```python
from build123d import *

# Parameters (mm, degrees)
SKETCH2_W           = 100
SKETCH2_H           = 50
BOSS_EXTRUDE1_DEPTH = 25
CUT_EXTRUDE1_DEPTH  = 9
CUT_EXTRUDE2_DEPTH  = 6.4
SKETCH8_W           = 6
SKETCH8_H           = 6
CUT_EXTRUDE3_DEPTH  = 6
SKETCH9_W           = 5
SKETCH9_H           = 5
CUT_EXTRUDE4_DEPTH  = 5


with BuildPart() as part:
    # Sketch2 → Boss-Extrude1 (new body)
    with BuildSketch(Plane(origin=(0, 0, 0), x_dir=(1, 0, 0), z_dir=(0, 1, 0))):
        Rectangle(SKETCH2_W, SKETCH2_H)
    extrude(amount=-BOSS_EXTRUDE1_DEPTH)

    # Sketch3 → Cut-Loft4 section 0
    with BuildSketch(Plane(origin=(0, 0, 0), x_dir=(1, 0, 0), z_dir=(0, 1, 0))):
        with BuildLine():
            Line((-45, 20), (45, 20))
            Line((45, 20), (45, -20))
            Line((45, -20), (-45, -20))
            Line((-45, -20), (-45, 20))
        make_face()
    # Sketch4 → Cut-Loft4 section 1
    with BuildSketch(Plane.XZ.offset(25)):
        with BuildLine():
            Line((-5, 5), (5, 5))
            Line((5, 5), (5, -5))
            Line((5, -5), (-5, -5))
            Line((-5, -5), (-5, 5))
        make_face()
    loft(mode=Mode.SUBTRACT)

    # Sketch5 → Cut-Extrude1 (cut)
    with BuildSketch(Plane(origin=(0, 0, -25), x_dir=(-1, 0, 0), z_dir=(0, 0, -1))):
        Polygon((0, -8), (3.2, -8), (3.2, -25), (-3.2, -25), (-3.2, -8), align=None)
    extrude(amount=-CUT_EXTRUDE1_DEPTH, mode=Mode.SUBTRACT)

    # Sketch6 → Cut-Extrude2 (cut)
    with BuildSketch(Plane(origin=(-3.2, 0, 0), x_dir=(0, 0, -1), z_dir=(1, 0, 0))):
        Polygon((16, -25), (5.785369477, -25), (16, -8), align=None)
    extrude(amount=CUT_EXTRUDE2_DEPTH, mode=Mode.SUBTRACT)

    # Sketch8 → Cut-Extrude3 (cut)
    with BuildSketch(Plane.XZ.offset(25)):
        with Locations((-45, 20)):
            Rectangle(SKETCH8_W, SKETCH8_H)
        with Locations((45, 20)):
            Rectangle(SKETCH8_W, SKETCH8_H)
    extrude(amount=-CUT_EXTRUDE3_DEPTH, mode=Mode.SUBTRACT)

    # Sketch9 → Cut-Extrude4 (cut)
    with BuildSketch(Plane(origin=(0, 0, 0), x_dir=(1, 0, 0), z_dir=(0, 1, 0))):
        with Locations((47.5, -22.5)):
            Rectangle(SKETCH9_W, SKETCH9_H)
        with Locations((-47.5, -22.5)):
            Rectangle(SKETCH9_W, SKETCH9_H)
        with Locations((-47.5, 22.5)):
            Rectangle(SKETCH9_W, SKETCH9_H)
        with Locations((47.5, 22.5)):
            Rectangle(SKETCH9_W, SKETCH9_H)
    extrude(amount=-CUT_EXTRUDE4_DEPTH, mode=Mode.SUBTRACT)


solid = part.part
```
Build history of the part. All positions in model axes, mm. A direction names the side the tool comes from. Coordinates: 2 decimals unless noted, no trailing zeros. Order: outer loops, then holes, each group sorted by start corner. A loop starts at its lowest first (then second) coordinate and runs counter-clockwise, first axis right, second up. Notation, with made-up numbers: (66, 7.25) -> (118, 7.25) arc R9 ccw to (118, 22.25) -> close; hole circle Ø2 at (57.25, 35). An arc over 180 degrees is marked (long way). Answer in a Markdown table with one row per item. Add a question column.
Q1. Wall check: line 1 along X through (y, z) = (-23.25, 21.5); line 2 along X through (y, z) = (-5.25, 14.5); line 3 along X through (y, z) = (-1.75, 20.5). Give the ranges that are in metal, low to high. Write a range as [from, to].
Q2. Mould opens along Z. For faces 1 (the face through (-45, -22, 17)), 2 (the face through (47, -5, -23)), 3 (the face through (45, -22, 23)), 4 (the face through (-1, -7, -25)) say: +Z half, -Z half, draft (parallel to the pull), parting line (faces both ways), or undercut.
Q3. Band-saw the part on A-A, the plane z = -21. List the corners of the cut face in (x, y), then the cut area to 3 significant figures.
Q4. Which spindle directions (+Z, -Z, +X, -X, +Y, -Y) get a long thin tool onto all of the face, cutting with end or side? Do faces 5 (the face through (-48, -5, -23)), 6 (the face through (47, -5, 22)), 7 (the face through (-3.2, -16, -18)). Say none if no direction does.
Q5. Band-saw the part on B-B, the plane y = -20. Give the number of separate pieces and of enclosed holes in the cut face, then the cut area to 3 significant figures.
Q6. Drop flat-ended pins along their axis: pin 1 (5.5 mm diameter, centred on y = -2, z = -23.5, fed in from +X); pin 2 (2.5 mm diameter, centred on x = -48.5, y = -1.5, fed in from -Z); pin 3 (4 mm diameter, centred on x = -2.5, z = -15, fed in from +Y). Give the stop position or say it passes through.
Answers follow:
| question | item | result |
|---|---|---|
| 1 | line 1 | [-50, -48], [-42, 42], [48, 50] |
| 1 | line 2 | [-50, -36.6], [36.6, 50] |
| 1 | line 3 | [-45, 45] |
| 2 | face 1 | undercut |
| 2 | face 2 | draft |
| 2 | face 3 | undercut |
| 2 | face 4 | -Z half |
| 3 | outline | (-50, -25) -> (-3.2, -25) -> (-3.2, -8) -> (3.2, -8) -> (3.2, -25) -> (50, -25) -> (50, -5) -> (45, -5) -> (45, 0) -> (-45, 0) -> (-45, -5) -> (-50, -5) -> close |
| 3 | area | 2,340 mm^2 |
| 4 | face 5 | -Z, -X, +Y |
| 4 | face 6 | +Z, +X, +Y |
| 4 | face 7 | -Z, -Y |
| 5 | separate pieces | 1 |
| 5 | enclosed holes | 3 |
| 5 | area | 4,410 mm^2 |
| 6 | pin 1 | x = 45 |
| 6 | pin 2 | z = -20 |
| 6 | pin 3 | y = -5 |
